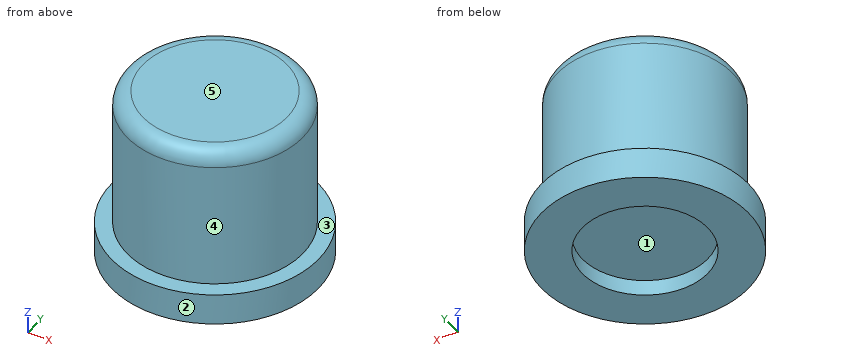
from build123d import *

# Parameters (mm, degrees)
SKETCH_1_R          = 2.8
EXTRUDE_1_DEPTH     = 5.5
SKETCH_2_R          = 3.3
EXTRUDE_2_DEPTH     = 1
SKETCH_3_R          = 2
CUT_EXTRUDE_1_DEPTH = 0.5
FILLET_1_R          = 0.5


with BuildPart() as part:
    # 草图1 → 凸台-拉伸1 (new body)
    with BuildSketch(Plane.XY):
        Circle(SKETCH_1_R)
    extrude(amount=EXTRUDE_1_DEPTH)

    # 草图2 → 凸台-拉伸2 (add)
    with BuildSketch(Plane(origin=(0, 0, 0), x_dir=(-1, 0, 0), z_dir=(0, 0, -1))):
        Circle(SKETCH_2_R)
    extrude(amount=-EXTRUDE_2_DEPTH)

    # 草图3 → 切除-拉伸1 (cut)
    with BuildSketch(Plane(origin=(0, 0, 0), x_dir=(-1, 0, 0), z_dir=(0, 0, -1))):
        Circle(SKETCH_3_R)
    extrude(amount=-CUT_EXTRUDE_1_DEPTH, mode=Mode.SUBTRACT)

    # 圆角1
    fillet_1_edges = [part.edges().sort_by_distance(p)[0] for p in [
        (-2.8, 0, 5.5),
    ]]
    fillet(fillet_1_edges, radius=FILLET_1_R)


solid = part.part
Build history of the part. All positions in model axes, mm. Face numbers are marked on the shaded views. A direction names the side the tool comes from. Round coordinates to 2 decimals unless told otherwise and drop trailing zeros. Loops run counter-clockwise (first coordinate to the right, second up) from the corner with the lowest first, then second, coordinate; pieces in that order, holes last. Notation, with made-up numbers: (-37.5, 78) -> (9.5, 78) arc R10 cw to (9.5, 89) -> close; hole circle Ø6 at (40.5, 52). An arc over 180 degrees is marked (long way). One line per item, written item: value. Start each with the question number.
Q1. Probe line 1 along Y through (x, z) = (0, 0.35); line 2 along Z through (x, y) = (-1.5, 0.25); line 3 along Z through (x, y) = (2.5, 2). List the from-to ranges inside material, lowest first.
Q2. Cut at D-D on z = 0.75. List the corners of the cut face in (x, y).
Q3. Cut at A-A on x = 0. List the corners of the cut face in (y, z).
Q4. Cut at C-C on z = 4.6. List the corners of the cut face in (x, y).
Q5. Drop flat-ended pins along their axis: pin 1 Ø2 at (x, z) = (1, 1.5) entering from -Y; pin 2 Ø2 at (x, z) = (2, 4) entering from -Y; pin 3 Ø1.5 at (x, y) = (-1, 0) entering from -Z. Give the stop position or say it passes through.
Q6. Two-plate mould, pull along X, no slides. Class the marked faces 1, 2 and 3: released by +X, released by -X, zero draft, split by the parting line, or undercut.
Q7. 3-axis set-ups, long thin cutter, end or side, ignore diameter. For the marked faces 4 and 5: which of +Z, -Z, +X, -X, +Y, -Y reach the whole face in a straight line?
Computed:
1. line 1: -3.3 to -2, 2 to 3.3
1. line 2: 0.5 to 5.5
1. line 3: 0 to 1
2. outline: circle Ø6.6 at (0, 0)
3. outline: (-3.3, 0) -> (-2, 0) -> (-2, 0.5) -> (2, 0.5) -> (2, 0) -> (3.3, 0) -> (3.3, 1) -> (2.8, 1) -> (2.8, 5) arc R0.5 ccw to (2.3, 5.5) -> (-2.3, 5.5) arc R0.5 ccw to (-2.8, 5) -> (-2.8, 1) -> (-3.3, 1) -> close
4. outline: circle Ø5.6 at (0, 0)
5. pin 1: y = -3.3
5. pin 2: y = -2.62
5. pin 3: z = 0.5
6. face 1: undercut
6. face 2: split by the parting line
6. face 3: zero draft
7. face 4: +Z
7. face 5: +Z, +X, -X, +Y, -Y
